Geometry check sheet. Reference: the model listing, model coordinates, mm. A direction names the side the tool comes from. Give positions to 0.01 mm unless a question says otherwise; leave off trailing zeros. Loops run counter-clockwise (first coordinate to the right, second up) from the corner with the lowest first, then second, coordinate; pieces in that order, holes last.
1. Cross-section at B-B, the plane z = 12.7. Record the cut outline in (x, y) (3 decimals).
2. Go/stop test with flat-tipped pins: pin 1 Ø4 at (x, z) = (12.7, 12.7) entering from +Y; pin 2 Ø8.5 at (y, z) = (41.275, 12.7) entering from +X (3 decimals); pin 3 Ø2 at (x, y) = (3.5, 32) entering from -Z; pin 4 Ø4 at (x, z) = (14, 4) entering from +Y (3 decimals). Record where each tip stops, or that it passes through.
3. Release check for a two-part mould opening along Y. For faces 1 (the cylindrical face through (1.57, 18.05, 14.09)), 2 (the flat face through (0, 26, 13)), 3 (the flat face through (12.5, 0, 9.7)) record: +Y half, -Y half, draft (parallel to the pull), parting line (faces both ways), or undercut.
4. Cross-section at A-A, the plane x = 12.7. Record the cut outline in (y, z) (3 decimals).
5. Cross-section at C-C, the plane z = 7. Record the cut outline in (x, y) (3 decimals).
6. Tool access check on faces 4 (the flat face through (17, 3.175, 13)), 5 (the flat face through (25.4, 2, 13)). Record the directions out of +Z, -Z, +X, -X, +Y, -Y that give a thin tool (end or side, any length) a straight path to the whole face; none if there is none.
7. Material ranges on L1, parallel to Y at x = 2.5, z = 12.7; L2, parallel to X at y = 1.7, z = 12.7, recorded low to high.
8. Cross-section at D-D, the plane y = 8. Record the cut outline in (x, z) (3 decimals), plus the area to 3 significant figures.
Autodesk Inventor part; units mm, degrees
ref_plane "YZ Plane" through (0, 0, 0) normal (1, 0, 0) x (0, 1, 0)
ref_plane "XZ Plane" through (0, 0, 0) normal (0, 1, 0) x (-1, 0, 0)
ref_plane "XY Plane" through (0, 0, 0) normal (0, 0, 1) x (1, 0, 0)
sketch "Sketch1" plane through (0, 0, 0) normal (0, 0, 1) x (1, 0, 0)
  line L0 (0, 0) -> (3.175, 0)
  line L1 (3.175, 0) -> (3.175, 50.8)
  line L2 (3.175, 50.8) -> (0, 50.8)
  line L3 (0, 50.8) -> (0, 0)
  line L4 (0, 0) -> (25.4, 0)
  line L5 (25.4, 0) -> (25.4, 3.175)
  line L6 (25.4, 3.175) -> (0, 3.175)
  line L7 (0, 3.175) -> (0, 0)
  dimension "d0" = 3.175
  dimension "d1" = 50.8
  dimension "d2" = 25.4
  dimension "d3" = 3.175
extrude "Extrusion1" add sketch "Sketch1" along normal blind 25.4
sketch "Sketch2" plane through (0, 0, 0) normal (-1, 0, 0) x (0, 0, 1)
  line L0 (0, 0) -> (25.4, 0)
  line L1 (12.7, 0) -> (12.7, 15.875)
  line L2 (12.7, 15.875) -> (12.7, 41.275)
  circle A0 centre (12.7, 41.275) radius 2.5797
  circle A1 centre (12.7, 15.875) radius 2.5797
  dimension "d6" = 15.875
  dimension "d7" = 25.4
  dimension "d8" = 5.1594
  dimension "d9" = 5.1594
extrude "Extrusion2" cut sketch "Sketch2" against normal blind 25.4
sketch "Sketch3" plane through (0, 0, 0) normal (0, -1, 0) x (1, 0, 0)
  line L0 (0, 0) -> (0, 25.4)
  line L1 (0, 12.7) -> (12.7, 12.7)
  circle A0 centre (12.7, 12.7) radius 2.5797
  dimension "d12" = 12.7
  dimension "d13" = 5.1594
extrude "Extrusion3" cut sketch "Sketch3" against normal blind 25.4
properties part number "1x2 L Bracket"
Result:
1. outline: (0, 0) - (10.12, 0) - (10.12, 3.175) - (3.175, 3.175) - (3.175, 13.295) - (0, 13.295) - close; (0, 18.455) - (3.175, 18.455) - (3.175, 38.695) - (0, 38.695) - close; (0, 43.855) - (3.175, 43.855) - (3.175, 50.8) - (0, 50.8) - close; (15.28, 0) - (25.4, 0) - (25.4, 3.175) - (15.28, 3.175) - close
2. pin 1: passes through
2. pin 2: stops at x = 3.175
2. pin 3: stops at z = 0
2. pin 4: stops at y = 3.175
3. face 1: undercut
3. face 2: draft
3. face 3: -Y half
4. outline: (0, 0) - (3.175, 0) - (3.175, 10.12) - (0, 10.12) - close; (0, 15.28) - (3.175, 15.28) - (3.175, 25.4) - (0, 25.4) - close
5. outline: (0, 0) - (25.4, 0) - (25.4, 3.175) - (3.175, 3.175) - (3.175, 50.8) - (0, 50.8) - close
6. face 4: +Z, -Z, +X, +Y
6. face 5: +Z, -Z, +X, +Y, -Y
7. L1: y = 0 to 13.3, 18.45 to 38.7, 43.85 to 50.8
7. L2: x = 0 to 10.12, 15.28 to 25.4
8. outline: (0, 0) - (3.175, 0) - (3.175, 25.4) - (0, 25.4) - close
8. area: 80.6 mm2
